```python
from build123d import *

# Parameters (mm, degrees)
SKETCH1_W           = 80
SKETCH1_H           = 60
BOSS_EXTRUDE1_DEPTH = 40
SKETCH2_W           = 60
SKETCH2_H           = 7.368056933
CUT_EXTRUDE1_DEPTH  = 83.462112512
BOSS_EXTRUDE2_DEPTH = 20
SKETCH5_R           = 7
CUT_EXTRUDE2_DEPTH  = 77.085478247
SKETCH6_R           = 25
CUT_EXTRUDE3_DEPTH  = 5
SKETCH7_R           = 20
BOSS_EXTRUDE3_DEPTH = 55
SKETCH8_R           = 14
CUT_EXTRUDE4_DEPTH  = 106.422957652
SKETCH11_W          = 14
SKETCH11_H          = 14
CUT_EXTRUDE5_DEPTH  = 10


with BuildPart() as part:
    # Sketch1 → Boss-Extrude1 (new body)
    with BuildSketch(Plane.XY):
        Rectangle(SKETCH1_W, SKETCH1_H)
    extrude(amount=-BOSS_EXTRUDE1_DEPTH)

    # Sketch2 → Cut-Extrude1 (cut, through all)
    with BuildSketch(Plane(origin=(0, 30, 0), x_dir=(1, 0, 0), z_dir=(0, 1, 0))):
        with Locations((0, 3.684028467)):
            Rectangle(SKETCH2_W, SKETCH2_H)
    extrude(amount=-CUT_EXTRUDE1_DEPTH, mode=Mode.SUBTRACT)

    # Sketch4 → Boss-Extrude2 (add)
    with BuildSketch(Plane.XY):
        with BuildLine():
            Line((40, -14), (53, -14))
            ThreePointArc((53, -14), (67, 0), (53, 14))
            Line((53, 14), (40, 14))
            Line((40, 14), (40, -14))
        make_face()
    boss_extrude2 = extrude(amount=-BOSS_EXTRUDE2_DEPTH)

    # Sketch5 → Cut-Extrude2 (cut, through all)
    with BuildSketch(Plane(origin=(0, 0, -20), x_dir=(-1, 0, 0), z_dir=(0, 0, -1))):
        with Locations((-53, 0)):
            Circle(SKETCH5_R)
    cut_extrude2 = extrude(amount=-CUT_EXTRUDE2_DEPTH, mode=Mode.SUBTRACT)

    # Mirror1: Boss-Extrude2, Cut-Extrude2 across plane
    add(boss_extrude2.mirror(Plane(origin=(0, 0, 0), x_dir=(0, 0, 1), z_dir=(1, 0, 0))))
    add(cut_extrude2.mirror(Plane(origin=(0, 0, 0), x_dir=(0, 0, 1), z_dir=(1, 0, 0))), mode=Mode.SUBTRACT)

    # Sketch6 → Cut-Extrude3 (cut)
    with BuildSketch(Plane.XZ.offset(30)):
        with Locations((0, -40)):
            Circle(SKETCH6_R)
    cut_extrude3 = extrude(amount=-CUT_EXTRUDE3_DEPTH, mode=Mode.SUBTRACT)

    # Mirror2: Cut-Extrude3 across plane
    add(cut_extrude3.mirror(Plane.ZX), mode=Mode.SUBTRACT)

    # Sketch7 → Boss-Extrude3 (add, through all)
    with BuildSketch(Plane.XZ.offset(25)):
        with Locations(Location((0, -40, 0), (0, 0, 270))):
            Circle(SKETCH7_R)
    extrude(amount=-BOSS_EXTRUDE3_DEPTH)

    # Sketch8 → Cut-Extrude4 (cut, through all)
    with BuildSketch(Plane.XZ.offset(25)):
        with Locations(Location((0, -40, 0), (0, 0, 270))):
            Circle(SKETCH8_R)
    extrude(amount=-CUT_EXTRUDE4_DEPTH, mode=Mode.SUBTRACT)

    # Sketch11 → Cut-Extrude5 (cut)
    with BuildSketch(Plane.XY.offset(-60)):
        with Locations((0, 5)):
            Rectangle(SKETCH11_W, SKETCH11_H)
    extrude(amount=CUT_EXTRUDE5_DEPTH, mode=Mode.SUBTRACT)


solid = part.part
```
The listing builds one solid part. Answer for the finished solid, in the listing's coordinates (mm). A direction names the side the tool comes from. Give positions to 0.01 mm unless a question says otherwise; leave off trailing zeros. Loops run counter-clockwise (first coordinate to the right, second up) from the corner with the lowest first, then second, coordinate; pieces in that order, holes last. Notation, with made-up numbers: (-37, 24) - (7, 24) arc R28 cw to (7, 52) - close; hole circle Ø1 at (1, 81.25). An arc over 180 degrees is marked (long way). Answer as CSV lines item,"result". Start each with the question number.
Item 1: A cutting plane is placed at B-B on y = 0. Determine the outline of the cut face in (x, z) (3 decimals).
Item 2: A cutting plane is placed at A-A on x = 0. Determine the outline of the cut face in (y, z), then the cut area to 3 significant figures.
Item 3: A cutting plane is placed at C-C on z = -35.5. Determine the outline of the cut face in (x, y).
Item 4: Each of these flat-tipped pins is pushed along its axis until it touches: pin 1 (2 mm diameter, centred on y = 24, z = -36.5, fed in from -X); pin 2 (6 mm diameter, centred on x = -27, y = 10.5, fed in from -Z); pin 3 (10.5 mm diameter, centred on x = -46, z = -6.5, fed in from +Y); pin 4 (10 mm diameter, centred on x = -3.5, z = -37, fed in from -Y). Where does it stop, or does it pass through?
Item 5: Find the intervals of material crossed by line 1 (Y direction, x = -53, z = -11); line 2 (Z direction, x = 27.5, y = 25); line 3 (X direction, y = -25, z = -12), in increasing order. Write a range as from..to.
Item 6: A cutting plane is placed at D-D on y = 16. Determine the outline of the cut face in (x, z), then the cut area to 3 significant figures.
Item 7: For faces 1 (the face through (0, 12, -56)), 2 (the face through (-46, -14, -10)), 3 (the face through (0.55, 27.535, -15.006)), 4 (the face through (56.3, 6.4, -20)), determine the directions among +Z, -Z, +X, -X, +Y, -Y from which every point of the face is accessible in a straight line to the end or side of a thin tool.
Item 8: The mould has two halves that part along X. Classify faces 5 (the face through (14, 30, -44)), 6 (the face through (0.55, -27.535, -15.006)), 7 (the face through (-67, 0, -10)): +X half, -X half, draft (parallel to the pull), parting line (faces both ways), or undercut.
Found:
1,outline,"(-67, -20) - (-60, -20) - (-60, 0) - (-67, 0) - close; (-46, -20) - (-40, -20) - (-40, -40) - (-20, -40) arc R20 ccw to (-7, -58.735) - (-7, -52.124) arc R14 cw (long way) to (7, -52.124) - (7, -58.735) arc R20 ccw to (20, -40) - (40, -40) - (40, -20) - (46, -20) - (46, 0) - (30, 0) - (30, -7.368) - (-30, -7.368) - (-30, 0) - (-46, 0) - close; (60, -20) - (67, -20) - (67, 0) - (60, 0) - close"
2,outline,"(-30, -15) - (-25, -15) - (-25, -26) - (30, -26) - (30, -20) - (25, -20) - (25, -15) - (30, -15) - (30, -7.37) - (-30, -7.37) - close; (-25, -60) - (-2, -60) - (-2, -54) - (-25, -54) - close; (12, -60) - (30, -60) - (30, -54) - (12, -54) - close"
2,area,"1,280 mm^2"
3,outline,"(-40, -30) - (-24.59, -30) - (-24.59, -25) - (-13.26, -25) - (-13.26, 30) - (-19.49, 30) - (-19.49, 25) - (-24.59, 25) - (-24.59, 30) - (-40, 30) - close; (13.26, -25) - (24.59, -25) - (24.59, -30) - (40, -30) - (40, 30) - (24.59, 30) - (24.59, 25) - (19.49, 25) - (19.49, 30) - (13.26, 30) - close"
4,pin 1,"stops at x = -40"
4,pin 2,"stops at z = -40"
4,pin 3,"stops at y = 14"
4,pin 4,"passes through"
5,line 1,"y = -14..-7, 7..14"
5,line 2,"z = -40..-7.37"
5,line 3,"x = -40..40"
6,outline,"(-40, -40) - (-20, -40) arc R20 ccw to (20, -40) - (40, -40) - (40, 0) - (30, 0) - (30, -7.37) - (-30, -7.37) - (-30, 0) - (-40, 0) - close; hole circle Ø28 at (0, -40)"
6,area,"2,770 mm^2"
7,face 1,"-Z"
7,face 2,"+Z, -Z, -X, -Y"
7,face 3,"+Y"
7,face 4,"-Z, +X, +Y, -Y"
8,face 5,"draft"
8,face 6,"undercut"
8,face 7,"-X half"
